from build123d import *

# Parameters (mm, degrees)
BOSS_EXTRUDE1_DEPTH = 100


with BuildPart() as part:
    # Sketch3 → Boss-Extrude1 (new body)
    with BuildSketch(Plane(origin=(0, 0, 0), x_dir=(0, 0, -1), z_dir=(1, 0, 0))):
        with BuildLine():
            Line((-5.515685425, 6.807463915), (-2.601114729, 3.892893219))
            ThreePointArc((-2.601114729, 3.892893219), (-2.27669138, 3.676120467), (-1.894007948, 3.6))
            Line((-1.894007948, 3.6), (0, 3.6))
            Line((0, 3.6), (0, 2.15))
            ThreePointArc((0, 2.15), (-1.52027958, 1.52027958), (-2.15, 0))
            Line((-2.15, 0), (-3.6, 0))
            Line((-3.6, 0), (-3.6, 1.894007948))
            ThreePointArc((-3.6, 1.894007948), (-3.676120467, 2.27669138), (-3.892893219, 2.601114729))
            Line((-3.892893219, 2.601114729), (-6.807463915, 5.515685425))
            ThreePointArc((-6.807463915, 5.515685425), (-7.679296086, 5.689103626), (-8.17314934, 4.95))
            Line((-8.17314934, 4.95), (-8.17314934, 2.7))
            ThreePointArc((-8.17314934, 2.7), (-8.231727984, 2.558578644), (-8.37314934, 2.5))
            Line((-8.37314934, 2.5), (-9.4, 2.5))
            ThreePointArc((-9.4, 2.5), (-9.824264069, 2.675735931), (-10, 3.1))
            Line((-10, 3.1), (-10, 8.5))
            ThreePointArc((-10, 8.5), (-9.560660172, 9.560660172), (-8.5, 10))
            Line((-8.5, 10), (-3.1, 10))
            ThreePointArc((-3.1, 10), (-2.675735931, 9.824264069), (-2.5, 9.4))
            Line((-2.5, 9.4), (-2.5, 8.37314934))
            ThreePointArc((-2.5, 8.37314934), (-2.558578644, 8.231727984), (-2.7, 8.17314934))
            Line((-2.7, 8.17314934), (-4.95, 8.17314934))
            ThreePointArc((-4.95, 8.17314934), (-5.689103626, 7.679296086), (-5.515685425, 6.807463915))
        make_face()
    extrude(amount=-BOSS_EXTRUDE1_DEPTH)

    # Mirror1: part across plane


with BuildPart() as part_1:
    add(part.part)
    add(part.part.mirror(Plane.ZX))

    # Mirror2: part across plane


with BuildPart() as part_2:
    add(part_1.part)
    add(part_1.part.mirror(Plane.XY))


solid = part_2.part
The listing builds one solid part. Answer for the finished solid, in the listing's coordinates (mm). A direction names the side the tool comes from. Give positions to 0.01 mm unless a question says otherwise; leave off trailing zeros. Write each loop counter-clockwise with the first axis right and the second up, starting at its lowest first coordinate (ties: lowest second). Pieces come first, ordered by that corner, then holes.
1) For a pull along Z with two mould halves and no side action, classify faces 6 (the face through (-100, -2.4, 0.1)), 7 (the face through (-49, -6, 10)), 8 (the face through (-49, 3.6, 0)) as pulls with the +Z half, pulls with the -Z half, needs draft (parallel to the pull), parting line crosses it, or undercut.
2) Find the intervals of material crossed by L1, parallel to Y at x = -7.5, z = -1; L2, parallel to Z at x = -34, y = -7.25; L3, parallel to Z at x = -70, y = 0, in increasing order.
3) Given P1, Ø0.5, axis at x = -34, y = 9, coming from the -Z side; P2, Ø0.8, axis at x = -49, z = -9, coming from the -Y side; P3, Ø1.1, axis at x = -58, y = -0.5, coming from the +Z side, each flat-ended and moving along its own axis, determine where each tip first touches the part or whether it passes through.
4) A tool of negligible diameter and unlimited length cuts with its end or side. For faces 1 (the face through (-49, -3.6, 0)), 2 (the face through (-49, 0, 3.6)), 3 (the face through (-49, -4, -8.173)), 4 (the face through (-49, -6, -10)), 5 (the face through (-49, -10, -6)), from which of +Z, -Z, +X, -X, +Y, -Y can it reach the whole face along a straight path? Write none if from no direction.
5) Section A-A (y = 1) is taken. Write down the section's boundary in (x, z).
Response:
1. face 6: needs draft
1. face 7: pulls with the +Z half
1. face 8: undercut
2. L1: y = -3.6 to -1.9, 1.9 to 3.6
2. L2: z = -10 to -5.74, 5.74 to 10
2. L3: z = -3.6 to -2.15, 2.15 to 3.6
3. P1: stops at z = -9.98
3. P2: stops at y = -10
3. P3: stops at z = 3.6
4. face 1: +X, -X, -Y
4. face 2: +Z, +X, -X
4. face 3: +X, -X
4. face 4: -Z, +X, -X, +Y, -Y
4. face 5: +Z, -Z, +X, -X, -Y
5. outline: (-100, -3.6) - (0, -3.6) - (0, -1.9) - (-100, -1.9) - close; (-100, 1.9) - (0, 1.9) - (0, 3.6) - (-100, 3.6) - close
